from build123d import *

# Parameters (mm, degrees)
ESQUISSE1_W             = 32
ESQUISSE1_H             = 40
BOSS_EXTRU_1_DEPTH      = 2
ESQUISSE2_W             = 2
ESQUISSE2_H             = 40
BOSS_EXTRU_2_DEPTH      = 28
CONG_1_R                = 20
ESQUISSE3_R             = 4
ENL_V_MAT_EXTRU_1_DEPTH = 30
ESQUISSE4_W             = 10.5
ESQUISSE4_H             = 10.5
ENL_V_MAT_EXTRU_2_DEPTH = 30
ESQUISSE5_W             = 1
ESQUISSE5_H             = 1
ESQUISSE5_W_2           = 10.5
ESQUISSE5_H_2           = 10.5
BOSS_EXTRU_5_DEPTH      = 1.5
ESQUISSE6_W             = 1
ESQUISSE6_H             = 10.5
BOSS_EXTRU_6_DEPTH      = 10.5
ESQUISSE7_R             = 2.5
ENL_V_MAT_EXTRU_3_DEPTH = 10.5
BOSS_EXTRU_7_START      = -30
ESQUISSE8_R             = 4
BOSS_EXTRU_7_DEPTH      = 30


with BuildPart() as part:
    # Esquisse1 → Boss.-Extru.1 (new body)
    with BuildSketch(Plane.XY):
        with Locations((-16, 20)):
            Rectangle(ESQUISSE1_W, ESQUISSE1_H)
    extrude(amount=BOSS_EXTRU_1_DEPTH)

    # Esquisse2 → Boss.-Extru.2 (add)
    with BuildSketch(Plane.XY.offset(2)):
        with Locations((-1, 20)):
            Rectangle(ESQUISSE2_W, ESQUISSE2_H)
    extrude(amount=BOSS_EXTRU_2_DEPTH)

    # Congé1
    cong_1_edges = [part.edges().sort_by_distance(p)[0] for p in [
        (-1, 40, 30),
        (-1, 0, 30),
    ]]
    fillet(cong_1_edges, radius=CONG_1_R - 0.0001)  # a hair under: the kernel refuses the full size

    # Esquisse3 → Enlèv. mat.-Extru.1 (cut)
    with BuildSketch(Plane(origin=(0, 0, 0), x_dir=(0, 0, -1), z_dir=(1, 0, 0))):
        with Locations(Location((-20.5, 20, 0), (0, 0, 90))):
            Circle(ESQUISSE3_R)
    extrude(amount=-ENL_V_MAT_EXTRU_1_DEPTH, mode=Mode.SUBTRACT)

    # Esquisse4 → Enlèv. mat.-Extru.2 (cut)
    with BuildSketch(Plane.XY.offset(2)):
        with Locations((-26.75, 34.75)):
            Rectangle(ESQUISSE4_W, ESQUISSE4_H)
        with Locations((-26.75, 5.25)):
            Rectangle(ESQUISSE4_W, ESQUISSE4_H)
    extrude(amount=-ENL_V_MAT_EXTRU_2_DEPTH, mode=Mode.SUBTRACT)

    # Esquisse5 → Boss.-Extru.5 (add)
    with BuildSketch(Plane.XY.offset(2)):
        with Locations((-21, 29)):
            Rectangle(ESQUISSE5_W, ESQUISSE5_H)
        with Locations((-26.75, 29)):
            Rectangle(ESQUISSE5_W_2, ESQUISSE5_H)
        with Locations((-21, 34.75)):
            Rectangle(ESQUISSE5_W, ESQUISSE5_H_2)
        with Locations((-21, 11)):
            Rectangle(ESQUISSE5_W, ESQUISSE5_H)
        with Locations((-21, 5.25)):
            Rectangle(ESQUISSE5_W, ESQUISSE5_H_2)
        with Locations((-26.75, 11)):
            Rectangle(ESQUISSE5_W_2, ESQUISSE5_H)
    extrude(amount=BOSS_EXTRU_5_DEPTH)

    # Esquisse6 → Boss.-Extru.6 (add)
    with BuildSketch(Plane.ZY.offset(21.5)):
        with Locations((3, 34.75)):
            Rectangle(ESQUISSE6_W, ESQUISSE6_H)
        with Locations((3, 5.25)):
            Rectangle(ESQUISSE6_W, ESQUISSE6_H)
    extrude(amount=BOSS_EXTRU_6_DEPTH)

    # Esquisse7 → Enlèv. mat.-Extru.3 (cut)
    with BuildSketch(Plane.XY.offset(3.5)):
        with Locations((-27, 35)):
            Circle(ESQUISSE7_R)
        with Locations((-27, 5)):
            Circle(ESQUISSE7_R)
    extrude(amount=-ENL_V_MAT_EXTRU_3_DEPTH, mode=Mode.SUBTRACT)

    # Esquisse8 → Boss.-Extru.7 (add)
    with BuildSketch(Plane.ZY.offset(2).offset(BOSS_EXTRU_7_START)):
        with Locations((20.5, 20)):
            Circle(ESQUISSE8_R)
    extrude(amount=BOSS_EXTRU_7_DEPTH)


solid = part.part
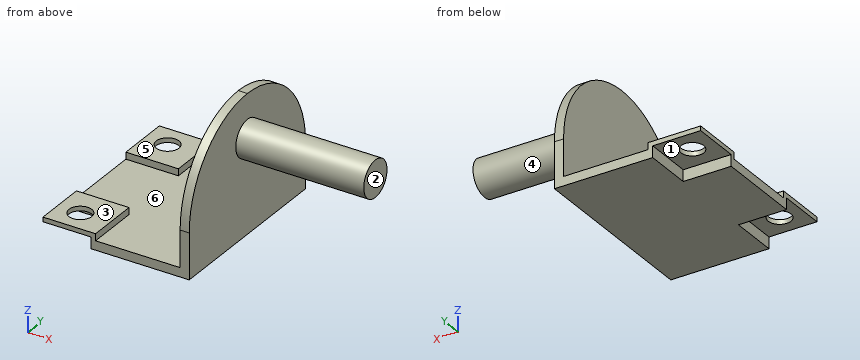
Design review of the part built by this model. Coordinates are the model's own, in mm. Face numbers are marked on the shaded views. A direction names the side the tool comes from. Give positions to 0.01 mm unless a question says otherwise; leave off trailing zeros. Order: outer loops, then holes, each group sorted by start corner. A loop starts at its lowest first (then second) coordinate and runs counter-clockwise, first axis right, second up. Notation, with made-up numbers: (4.25, 71.5) - (38.25, 71.5) arc R29 ccw to (38.25, 110.5) - close; hole circle Ø8 at (47.25, 88.5). An arc over 180 degrees is marked (long way). Use CSV: the item, a comma, the result in double quotes. Start each with the question number.
Q1. Draft analysis for pull direction Y (two halves, no side actions). For the marked faces 4, 5 and 6, state which applies: pulls with the +Y half, pulls with the -Y half, needs draft (parallel to the pull), parting line crosses it, or undercut.
Q2. For P1, Ø8, axis at x = -20.5, y = 36, coming from the +Z side; P2, Ø6, axis at y = 23, z = 9.5, coming from the -X side; P3, Ø2, axis at x = 22, z = 21, coming from the +Y side, all flat-tipped, find the tip position at first contact; note any pin that passes through.
Q3. Take a section at B-B (y = 35). State the section outline as (x, z) points.
Q4. Take a section at C-C (y = 22.5). State the section outline as (x, z) points, and give its area (3 significant figures).
Q5. Take a section at D-D (x = -5). State the section outline as (y, z) points.
Q6. For line 1 (Y direction, x = -27, z = 2.8); line 2 (X direction, y = 10, z = 4); line 3 (Z direction, x = -22, y = 18.5), list the stretches that pass through material, from the lowest coordinate up.
Q7. Take a section at A-A (x = -27). State the section outline as (y, z) points.
Q8. Machinability: for the marked faces 1, 2 and 3, which of the approach directions +Z, -Z, +X, -X, +Y, -Y give a long, thin tool a straight path to every point of the face, cutting with its end or side? Answer none if there is none.
Calculated:
1,face 4,"parting line crosses it"
1,face 5,"needs draft"
1,face 6,"undercut"
2,P1,"stops at z = 3.5"
2,P2,"stops at x = -2"
2,P3,"stops at y = 24"
3,outline,"(-32, 2.5) - (-29.5, 2.5) - (-29.5, 3.5) - (-32, 3.5) - close; (-24.5, 2.5) - (-21.5, 2.5) - (-21.5, 0) - (0, 0) - (0, 23.23) - (-2, 23.23) - (-2, 2) - (-20.5, 2) - (-20.5, 3.5) - (-24.5, 3.5) - close"
4,outline,"(-32, 0) - (0, 0) - (0, 17.38) - (28, 17.38) - (28, 23.62) - (0, 23.62) - (0, 29.84) - (-2, 29.84) - (-2, 2) - (-32, 2) - close"
4,area,"295 mm²"
5,outline,"(0, 0) - (40, 0) - (40, 2) - (0, 2) - close"
6,line 1,"y = 0 to 2.5, 7.5 to 11.5, 28.5 to 32.5, 37.5 to 40"
6,line 2,"x = -2 to 0"
6,line 3,"z = 0 to 2"
7,outline,"(0, 2.5) - (2.5, 2.5) - (2.5, 3.5) - (0, 3.5) - close; (7.5, 2.5) - (10.5, 2.5) - (10.5, 0) - (29.5, 0) - (29.5, 2.5) - (32.5, 2.5) - (32.5, 3.5) - (28.5, 3.5) - (28.5, 2) - (11.5, 2) - (11.5, 3.5) - (7.5, 3.5) - close; (37.5, 2.5) - (40, 2.5) - (40, 3.5) - (37.5, 3.5) - close"
8,face 1,"-Z, -X, +Y"
8,face 2,"+Z, -Z, +X, +Y, -Y"
8,face 3,"+Z, -X, +Y, -Y"
